```python
from build123d import *

# Parameters (mm, degrees)
ESTRUSIONE_ESTRUSIONE1_DEPTH = 600


with BuildPart() as part:
    # Schizzo1 → Estrusione-Estrusione1 (new body)
    with BuildSketch(Plane(origin=(0, 0, -600), x_dir=(-1, 0, 0), z_dir=(0, 0, -1))):
        with BuildLine():
            Line((-15, 13), (-15, -13))
            ThreePointArc((-15, -13), (-14.414213562, -14.414213562), (-13, -15))
            Line((-13, -15), (13, -15))
            ThreePointArc((13, -15), (14.414213562, -14.414213562), (15, -13))
            Line((15, -13), (15, -4))
            Line((15, -4), (13, -4))
            Line((13, -4), (13, -8.25))
            Line((13, -8.25), (9.664213562, -8.25))
            add(Edge.make_bspline(
                [(9.664213562, -8.25), (8.442809042, -7.028595479), (7.221404521, -5.807190958), (6, -4.585786438)],
                knots=[0, 0, 0, 0, 1, 1, 1, 1], degree=3))
            Line((6, -4.585786438), (6, -2.5))
            Line((6, -2.5), (5.750976629, -1.218885816))
            Line((5.750976629, -1.218885816), (5.933012788, -0.90358969))
            ThreePointArc((5.933012788, -0.90358969), (6, -0.653589753), (5.933012702, -0.403589838))
            Line((5.933012702, -0.403589838), (5.7, 0))
            Line((5.7, 0), (5.933012702, 0.403589838))
            ThreePointArc((5.933012702, 0.403589838), (5.982962913, 0.524180316), (6, 0.653589838))
            Line((6, 0.653589838), (6, 4.585786438))
            add(Edge.make_bspline(
                [(6, 4.585786438), (7.221404521, 5.807190958), (8.442809042, 7.028595479), (9.664213562, 8.25)],
                knots=[0, 0, 0, 0, 1, 1, 1, 1], degree=3))
            Line((9.664213562, 8.25), (13, 8.25))
            Line((13, 8.25), (13, 4))
            Line((13, 4), (15, 4))
            Line((15, 4), (15, 13))
            ThreePointArc((15, 13), (14.414213562, 14.414213562), (13, 15))
            Line((13, 15), (4, 15))
            Line((4, 15), (4, 13))
            Line((4, 13), (8.25, 13))
            Line((8.25, 13), (8.25, 9.664213562))
            add(Edge.make_bspline(
                [(8.25, 9.664213562), (7.028595479, 8.442809042), (5.807190958, 7.221404521), (4.585786438, 6)],
                knots=[0, 0, 0, 0, 1, 1, 1, 1], degree=3))
            Line((4.585786438, 6), (2.5, 6))
            Line((2.5, 6), (1.218885629, 5.750976592))
            Line((1.218885629, 5.750976592), (0.903589838, 5.933012702))
            ThreePointArc((0.903589838, 5.933012702), (0.653589838, 6), (0.403589838, 5.933012702))
            Line((0.403589838, 5.933012702), (0, 5.7))
            Line((0, 5.7), (-0.403589838, 5.933012702))
            ThreePointArc((-0.403589838, 5.933012702), (-0.524180316, 5.982962913), (-0.653589838, 6))
            Line((-0.653589838, 6), (-4.585786438, 6))
            add(Edge.make_bspline(
                [(-4.585786438, 6), (-5.807190958, 7.221404521), (-7.028595479, 8.442809042), (-8.25, 9.664213562)],
                knots=[0, 0, 0, 0, 1, 1, 1, 1], degree=3))
            Line((-8.25, 9.664213562), (-8.25, 13))
            Line((-8.25, 13), (-4, 13))
            Line((-4, 13), (-4, 15))
            Line((-4, 15), (-13, 15))
            ThreePointArc((-13, 15), (-14.414213562, 14.414213562), (-15, 13))
        make_face()
        with BuildLine():
            Line((12.349838066, 9.914583088), (11.34224826, 9.54785039))
            ThreePointArc((11.34224826, 9.54785039), (9.873470565, 9.873470565), (9.54785039, 11.34224826))
            Line((9.54785039, 11.34224826), (9.914583088, 12.349838066))
            ThreePointArc((9.914583088, 12.349838066), (13.043502884, 13.043502884), (12.349838066, 9.914583088))
        make_face(mode=Mode.SUBTRACT)
        with BuildLine():
            Line((-4.585786438, -6), (4.58, -6))
            add(Edge.make_bspline(
                [(4.58, -6), (5.73, -7.15), (6.88, -8.3), (8.03, -9.45)],
                knots=[0, 0, 0, 0, 1, 1, 1, 1], degree=3))
            Line((8.03, -9.45), (11.1, -9.45))
            Line((11.1, -9.45), (12.361944654, -9.919036981))
            ThreePointArc((12.361944654, -9.919036981), (13.194761433, -12.872897378), (10.127586207, -12.766543418))
            ThreePointArc((10.127586207, -12.766543418), (9.169403304, -12.336446483), (8.355281336, -13))
            Line((8.355281336, -13), (-8.25, -13))
            Line((-8.25, -13), (-8.25, -9.664213562))
            add(Edge.make_bspline(
                [(-8.25, -9.664213562), (-7.028595479, -8.442809042), (-5.807190958, -7.221404521), (-4.585786438, -6)],
                knots=[0, 0, 0, 0, 1, 1, 1, 1], degree=3))
        make_face(mode=Mode.SUBTRACT)
        with BuildLine():
            Line((-9.919036981, 12.361944654), (-9.45, 11.1))
            Line((-9.45, 11.1), (-9.45, 8.03))
            add(Edge.make_bspline(
                [(-9.45, 8.03), (-8.3, 6.88), (-7.15, 5.73), (-6, 4.58)],
                knots=[0, 0, 0, 0, 1, 1, 1, 1], degree=3))
            Line((-6, 4.58), (-6, -4.585786438))
            add(Edge.make_bspline(
                [(-6, -4.585786438), (-7.221404521, -5.807190958), (-8.442809042, -7.028595479), (-9.664213562, -8.25)],
                knots=[0, 0, 0, 0, 1, 1, 1, 1], degree=3))
            Line((-9.664213562, -8.25), (-13, -8.25))
            Line((-13, -8.25), (-13, 8.355281336))
            ThreePointArc((-13, 8.355281336), (-12.336446483, 9.169403304), (-12.766543418, 10.127586207))
            ThreePointArc((-12.766543418, 10.127586207), (-12.872897378, 13.194761433), (-9.919036981, 12.361944654))
        make_face(mode=Mode.SUBTRACT)
        with BuildLine():
            Line((-9.54785039, -11.34224826), (-9.914583088, -12.349838066))
            ThreePointArc((-9.914583088, -12.349838066), (-13.043502884, -13.043502884), (-12.349838066, -9.914583088))
            Line((-12.349838066, -9.914583088), (-11.34224826, -9.54785039))
            ThreePointArc((-11.34224826, -9.54785039), (-9.873470565, -9.873470565), (-9.54785039, -11.34224826))
        make_face(mode=Mode.SUBTRACT)
        with BuildLine():
            Line((4, 3.5), (4, 2))
            ThreePointArc((4, 2), (3.879005736, 1.673879391), (3.574581393, 1.505593673))
            ThreePointArc((3.574581393, 1.505593673), (3.295837094, 1.323326833), (3.251694243, 0.993219284))
            ThreePointArc((3.251694243, 0.993219284), (3.4, 0), (3.251694243, -0.993219284))
            ThreePointArc((3.251694243, -0.993219284), (3.295837094, -1.323326833), (3.574581393, -1.505593673))
            ThreePointArc((3.574581393, -1.505593673), (3.879005736, -1.673879391), (4, -2))
            Line((4, -2), (4, -3.5))
            ThreePointArc((4, -3.5), (3.853553391, -3.853553391), (3.5, -4))
            Line((3.5, -4), (2, -4))
            ThreePointArc((2, -4), (1.673879391, -3.879005736), (1.505593673, -3.574581393))
            ThreePointArc((1.505593673, -3.574581393), (1.323326833, -3.295837094), (0.993219284, -3.251694243))
            ThreePointArc((0.993219284, -3.251694243), (0, -3.4), (-0.993219284, -3.251694243))
            ThreePointArc((-0.993219284, -3.251694243), (-1.323326833, -3.295837094), (-1.505593673, -3.574581393))
            ThreePointArc((-1.505593673, -3.574581393), (-1.673879391, -3.879005736), (-2, -4))
            Line((-2, -4), (-3.5, -4))
            ThreePointArc((-3.5, -4), (-3.853553391, -3.853553391), (-4, -3.5))
            Line((-4, -3.5), (-4, -2))
            ThreePointArc((-4, -2), (-3.879005736, -1.673879391), (-3.574581393, -1.505593673))
            ThreePointArc((-3.574581393, -1.505593673), (-3.295837094, -1.323326833), (-3.251694243, -0.993219284))
            ThreePointArc((-3.251694243, -0.993219284), (-3.4, 0), (-3.251694243, 0.993219284))
            ThreePointArc((-3.251694243, 0.993219284), (-3.295837094, 1.323326833), (-3.574581393, 1.505593673))
            ThreePointArc((-3.574581393, 1.505593673), (-3.879005736, 1.673879391), (-4, 2))
            Line((-4, 2), (-4, 3.5))
            ThreePointArc((-4, 3.5), (-3.853553391, 3.853553391), (-3.5, 4))
            Line((-3.5, 4), (-2, 4))
            ThreePointArc((-2, 4), (-1.673879391, 3.879005736), (-1.505593673, 3.574581393))
            ThreePointArc((-1.505593673, 3.574581393), (-1.323326833, 3.295837094), (-0.993219284, 3.251694243))
            ThreePointArc((-0.993219284, 3.251694243), (0, 3.4), (0.993219284, 3.251694243))
            ThreePointArc((0.993219284, 3.251694243), (1.323326833, 3.295837094), (1.505593673, 3.574581393))
            ThreePointArc((1.505593673, 3.574581393), (1.673879391, 3.879005736), (2, 4))
            Line((2, 4), (3.5, 4))
            ThreePointArc((3.5, 4), (3.853553391, 3.853553391), (4, 3.5))
        make_face(mode=Mode.SUBTRACT)
    extrude(amount=-ESTRUSIONE_ESTRUSIONE1_DEPTH)


solid = part.part
```
Input: part model. Units: mm. Frame: model coordinates. A direction names the side the tool comes from. Coordinates: 2 decimals unless noted, no trailing zeros. Put each result on its own line as item: value. Start each with the question number.
1) Reachability of faces 1 (the face through (0, -15, -304)), 2 (the face through (6, 0, -304)) from +Z, -Z, +X, -X, +Y, -Y: full face, straight path, thin tool, end or side. Return the list, or none.
2) Mould query, pull axis X, two halves, no side actions, for faces 3 (the face through (4, 0, 0)), 4 (the face through (15, 0, -304)), 5 (the face through (0, -6, -304)). Classes: pulls with the +X half, pulls with the -X half, needs draft (parallel to the pull), parting line crosses it, or undercut.
3) Ray query, L1, parallel to X at y = 11.7, z = -228; L2, parallel to X at y = 3.5, z = -334; L3, parallel to X at y = -2, z = -26.5. Return the intervals inside material, ascending.
4) Contact query for flat-ended pins moving along their axis: pin 1 (8 mm diameter, centred on x = 2.5, z = -379, fed in from +Y); pin 2 (0.8 mm diameter, centred on x = -2.5, z = -202.5, fed in from +Y). Output: stop coordinate, or through.
5) Cut plane A-A (z = -150). State how many separate pieces and enclosed holes the cut face has, plus the area to 3 significant figures.
Resolved:
1. face 1: +Z, -Z, +X, -X, -Y
1. face 2: +Z, -Z
2. face 3: needs draft
2. face 4: pulls with the +X half
2. face 5: undercut
3. L1: x = -15 to -13.6, -9.68 to -8.25, 8.25 to 9.67, 13.6 to 15
3. L2: x = -6 to -4, -1.49 to 1.49, 4 to 6, 13 to 15
3. L3: x = -5.9 to -4, 4 to 6, 13 to 15
4. pin 1: stops at y = 15
4. pin 2: stops at y = 6
5. separate pieces: 1
5. enclosed holes: 5
5. area: 339 mm2
